Model file for the job. Use its own axes, mm. Round coordinates to 2 decimals unless told otherwise and drop trailing zeros. Loops run counter-clockwise (first coordinate to the right, second up) from the corner with the lowest first, then second, coordinate; pieces in that order, holes last. Notation, with made-up numbers: (-20.5, 42.25) - (-13.5, 42.25) arc R18 cw to (-13.5, 72.25) - close; hole circle Ø9 at (80, 75). An arc over 180 degrees is marked (long way). Answer as a JSON object with one key per item and string values.
from build123d import *

# Parameters (mm, degrees)
F0_R     = 5
F1_DEPTH = 1


with BuildPart() as f1:
    # F0 (on Top) → F1 (new body)
    with BuildSketch(Plane.XY):
        with BuildLine():
            Line((-12.4, -27), (-10, -29))
            Line((-10, -29), (-10, -23))
            ThreePointArc((-10, -23), (-9, -22), (-8, -23))
            Line((-8, -23), (-8, -41))
            ThreePointArc((-8, -41), (0, -49), (8, -41))
            Line((8, -41), (8, -23))
            ThreePointArc((8, -23), (9, -22), (10, -23))
            Line((10, -23), (10, -29))
            Line((10, -29), (12.4, -27))
            Line((12.4, -27), (12.4, -23))
            Line((12.4, -23), (13.9, -23))
            Line((13.9, -23), (13.9, 0))
            ThreePointArc((13.9, 0), (0, 13.9), (-13.9, 0))
            Line((-13.9, 0), (-13.9, -23))
            Line((-13.9, -23), (-12.4, -23))
            Line((-12.4, -23), (-12.4, -27))
        make_face()
        with Locations((0, -41)):
            Circle(F0_R, mode=Mode.SUBTRACT)
    extrude(amount=F1_DEPTH)


solid = f1.part
1) Slice it at D-D on y = 7.5. List the corners of the cut face in (x, z), then the cut area to 3 significant figures.
Values follow:
{"outline": "(-11.7, 0) - (11.7, 0) - (11.7, 1) - (-11.7, 1) - close", "area": "23.4 mm²"}
2) Two-plate mould, pull along Y, no slides. Class faces 1 (the cylindrical face through (0.306, 13.897, 0.493)), 2 (the cylindrical face through (2.688, -36.784, 0.493)), 3 (the flat face through (0, -10, 1)), 4 (the flat face through (11.2, -28, 0.5)): pulls with the +Y half, pulls with the -Y half, needs draft (parallel to the pull), parting line crosses it, or undercut.
Values follow:
{"face 1": "pulls with the +Y half", "face 2": "undercut", "face 3": "needs draft", "face 4": "pulls with the -Y half"}
3) Probe probe 1 along Y at (x, z) = (0, 0.5); probe 2 along Y at (x, z) = (-2, 0.3); probe 3 along Y at (x, z) = (-10.5, 0.6). List the from-to ranges inside material, lowest first.
Values follow:
{"probe 1": "-49 to -46, -36 to 13.9", "probe 2": "-48.75 to -45.58, -36.42 to 13.76", "probe 3": "-28.58 to 9.11"}
4) Slice it at C-C on x = 9. List the corners of the cut face in (y, z), then the cut area to 3 significant figures.
Values follow:
{"outline": "(-22, 0) - (10.59, 0) - (10.59, 1) - (-22, 1) - close", "area": "32.6 mm²"}
5) Slice it at A-A on z = 0.8. List the corners of the cut face in (x, y).
Values follow:
{"outline": "(-13.9, -23) - (-12.4, -23) - (-12.4, -27) - (-10, -29) - (-10, -23) arc R1 cw to (-8, -23) - (-8, -41) arc R8 ccw to (8, -41) - (8, -23) arc R1 cw to (10, -23) - (10, -29) - (12.4, -27) - (12.4, -23) - (13.9, -23) - (13.9, 0) arc R13.9 ccw to (-13.9, 0) - close; hole circle Ø10 at (0, -41)"}
6) Drop flat-ended pins along their axis: P1, Ø0.5, axis at x = 13, z = 0.5, coming from the -Y side; P2, Ø0.5, axis at y = -24, z = 0.5, coming from the -X side; P3, Ø6, axis at x = 0, y = -41, coming from the -Z side; P4, Ø0.5, axis at y = -26, z = 0.5, coming from the +X side. Give the stop position or say it passes through.
Values follow:
{"P1": "y = -23", "P2": "x = -12.4", "P3": "through", "P4": "x = 12.4"}
7) Slice it at B-B on y = -44. List the corners of the cut face in (x, z), then the cut area to 3 significant figures.
Values follow:
{"outline": "(-7.42, 0) - (-4, 0) - (-4, 1) - (-7.42, 1) - close; (4, 0) - (7.42, 0) - (7.42, 1) - (4, 1) - close", "area": "6.83 mm²"}
